from build123d import *

# Parameters (mm, degrees)
SKETCH1_R          = 41.5
MAIN_PLATE_DEPTH   = 20
SKETCH3_R          = 2.5
SKETCH3_R_2        = 25
MOMO_SPARKO_DEPTH  = 63.004032127
SKETCH4_W          = 90
SKETCH4_H          = 45
CUT_EXTRUDE1_DEPTH = 5.25


with BuildPart() as part:
    # Sketch1 → Main Plate (new body)
    with BuildSketch(Plane(origin=(0, 0, 0), x_dir=(1, 0, 0), z_dir=(0, 1, 0))):
        with Locations(Location((0, 0, 0), (0, 0, 270))):
            Circle(SKETCH1_R)
    extrude(amount=MAIN_PLATE_DEPTH)

    # Sketch3 → Momo - Sparko (cut, through all)
    with BuildSketch(Plane(origin=(0, 20, 0), x_dir=(1, 0, 0), z_dir=(0, 1, 0))):
        with Locations(Location((0, 35, 0), (0, 0, 270))):
            Circle(SKETCH3_R)
        with Locations(Location((0, 0, 0), (0, 0, 270))):
            Circle(SKETCH3_R_2)
        with Locations(Location((30.310889132, 17.5, 0), (0, 0, 270))):
            Circle(SKETCH3_R)
        with Locations(Location((30.310889132, -17.5, 0), (0, 0, 270))):
            Circle(SKETCH3_R)
        with Locations(Location((0, -35, 0), (0, 0, 270))):
            Circle(SKETCH3_R)
        with Locations(Location((-30.310889132, -17.5, 0), (0, 0, 270))):
            Circle(SKETCH3_R)
        with Locations(Location((-30.310889132, 17.5, 0), (0, 0, 270))):
            Circle(SKETCH3_R)
    extrude(amount=-MOMO_SPARKO_DEPTH, mode=Mode.SUBTRACT)

    # Sketch4 → Cut-Extrude1 (cut)
    with BuildSketch(Plane.XZ):
        Rectangle(SKETCH4_W, SKETCH4_H)
    extrude(amount=-CUT_EXTRUDE1_DEPTH, mode=Mode.SUBTRACT)


solid = part.part
The listing builds one solid part. Answer for the finished solid, in the listing's coordinates (mm). A direction names the side the tool comes from. Give positions to 0.01 mm unless a question says otherwise; leave off trailing zeros. Write each loop counter-clockwise with the first axis right and the second up, starting at its lowest first coordinate (ties: lowest second). Pieces come first, ordered by that corner, then holes. Notation, with made-up numbers: (44.5, 52) -> (101.5, 52) arc R15 ccw to (101.5, 75) -> close; hole circle Ø8 at (35, 75.25). An arc over 180 degrees is marked (long way). Use a Markdown table: item, result.
(1) Find the intervals of material crossed by probe 1 along X at (y, z) = (8.5, -17.5); probe 2 along Z at (x, y) = (-30.5, 11); probe 3 along X at (y, z) = (19.25, -20.5), in increasing order. Write a range as from..to.
Return value:
| item | result |
|---|---|
| probe 1 | -37.63..-32.81, -27.81..-17.85, 17.85..27.81, 32.81..37.63 |
| probe 2 | -28.14..-19.99, -15.01..15.01, 19.99..28.14 |
| probe 3 | -36.08..-14.31, 14.31..36.08 |
(2) Section A-A, the plane y = 4.25 is taken. Determine the outline of the cut face in (x, z).
Return value:
| item | result |
|---|---|
| outline | (-34.87, -22.5) arc R41.5 ccw to (34.87, -22.5) -> (10.9, -22.5) arc R25 cw to (-10.9, -22.5) -> close; (-34.87, 22.5) -> (-10.9, 22.5) arc R25 cw to (10.9, 22.5) -> (34.87, 22.5) arc R41.5 ccw to start; hole circle Ø5 at (0, -35); hole circle Ø5 at (0, 35) |
(3) Flat-ended cylindrical pins translate along their axes: P1, Ø3, axis at y = 10, z = -32.5, coming from the -X side; P2, Ø4, axis at x = -20.5, y = 2.5, coming from the +Z side; P3, Ø1, axis at x = 27, y = 14, coming from the +Z side. Find the tip coordinate at first contact, or state that the pin passes through.
Return value:
| item | result |
|---|---|
| P1 | x = -27.59 |
| P2 | z = 37.15 |
| P3 | z = 31.94 |
(4) Section B-B, the plane x = -22.5 is taken. Determine the outline of the cut face in (y, z).
Return value:
| item | result |
|---|---|
| outline | (0, -34.87) -> (20, -34.87) -> (20, -10.9) -> (5.25, -10.9) -> (5.25, -22.5) -> (0, -22.5) -> close; (0, 22.5) -> (5.25, 22.5) -> (5.25, 10.9) -> (20, 10.9) -> (20, 34.87) -> (0, 34.87) -> close |
(5) Section C-C, the plane z = 0 is taken. Determine the outline of the cut face in (x, y), then the cut area to 3 significant figures.
Return value:
| item | result |
|---|---|
| outline | (-41.5, 5.25) -> (-25, 5.25) -> (-25, 20) -> (-41.5, 20) -> close; (25, 5.25) -> (41.5, 5.25) -> (41.5, 20) -> (25, 20) -> close |
| area | 487 mm2 |
(6) For faces 4 (the cylindrical face through (-0.96, 10.14, -32.69)), 5 (the flat face through (-30, 5.25, 0)), determine the directions among +Z, -Z, +X, -X, +Y, -Y from which every point of the face is accessible in a straight line to the end or side of a thin tool.
Return value:
| item | result |
|---|---|
| face 4 | +Y, -Y |
| face 5 | +X, -X, -Y |
(7) Determine the mould class of faces 1 (the cylindrical face through (1.82, 9.86, -41.46)), 2 (the cylindrical face through (-32.75, 12.73, -18.04)), 3 (the flat face through (-18, 20, 18)) for opening direction X: released by +X, released by -X, zero draft, split by the parting line, or undercut.
Return value:
| item | result |
|---|---|
| face 1 | split by the parting line |
| face 2 | undercut |
| face 3 | zero draft |
(8) Section D-D, the plane x = 0 is taken. Determine the outline of the cut face in (y, z), then the cut area to 3 significant figures.
Return value:
| item | result |
|---|---|
| outline | (0, -41.5) -> (20, -41.5) -> (20, -37.5) -> (0, -37.5) -> close; (0, -32.5) -> (20, -32.5) -> (20, -25) -> (0, -25) -> close; (0, 25) -> (20, 25) -> (20, 32.5) -> (0, 32.5) -> close; (0, 37.5) -> (20, 37.5) -> (20, 41.5) -> (0, 41.5) -> close |
| area | 460 mm2 |
